from build123d import *

# Parameters (mm, degrees)
SKETCH2_W           = 50
SKETCH2_H           = 225
SKETCH2_W_2         = 30
SKETCH2_H_2         = 205
BOSS_EXTRUDE1_DEPTH = 25
SKETCH3_W           = 140
SKETCH3_H           = 305
SKETCH3_W_2         = 30
SKETCH3_H_2         = 205
BOSS_EXTRUDE2_DEPTH = 10
BOSS_EXTRUDE3_DEPTH = 150
BOSS_EXTRUDE4_START = 20
BOSS_EXTRUDE4_DEPTH = 5
LPATTERN1_COUNT     = 6
LPATTERN1_PITCH     = 22


with BuildPart() as part:
    # Sketch2 → Boss-Extrude1 (new body)
    with BuildSketch(Plane.XY):
        Rectangle(SKETCH2_W, SKETCH2_H)
        Rectangle(SKETCH2_W_2, SKETCH2_H_2, mode=Mode.SUBTRACT)
    extrude(amount=-BOSS_EXTRUDE1_DEPTH)

    # Sketch3 → Boss-Extrude2 (add)
    with BuildSketch(Plane.XY):
        with Locations((15, 0)):
            Rectangle(SKETCH3_W, SKETCH3_H)
        Rectangle(SKETCH3_W_2, SKETCH3_H_2, mode=Mode.SUBTRACT)
    extrude(amount=BOSS_EXTRUDE2_DEPTH)

    # Sketch4 → Boss-Extrude3 (add)
    with BuildSketch(Plane.XY.offset(10)):
        with BuildLine():
            Line((-30, 137.5), (65, 137.5))
            ThreePointArc((65, 137.5), (75.606601718, 133.106601718), (80, 122.5))
            Line((80, 122.5), (80, -122.5))
            ThreePointArc((80, -122.5), (75.606601718, -133.106601718), (65, -137.5))
            Line((65, -137.5), (-30, -137.5))
            ThreePointArc((-30, -137.5), (-40.606601718, -133.106601718), (-45, -122.5))
            Line((-45, -122.5), (-45, 122.5))
            ThreePointArc((-45, 122.5), (-40.606601718, 133.106601718), (-30, 137.5))
        make_face()
        with BuildLine():
            Line((-25, 122.5), (60, 122.5))
            ThreePointArc((60, 122.5), (63.535533906, 121.035533906), (65, 117.5))
            Line((65, 117.5), (65, -117.5))
            ThreePointArc((65, -117.5), (63.535533906, -121.035533906), (60, -122.5))
            Line((60, -122.5), (-25, -122.5))
            ThreePointArc((-25, -122.5), (-28.535533906, -121.035533906), (-30, -117.5))
            Line((-30, -117.5), (-30, 117.5))
            ThreePointArc((-30, 117.5), (-28.535533906, 121.035533906), (-25, 122.5))
        make_face(mode=Mode.SUBTRACT)
    extrude(amount=BOSS_EXTRUDE3_DEPTH)

    # Sketch5 → Boss-Extrude4 (add)
    with BuildSketch(Plane.XY.offset(10).offset(BOSS_EXTRUDE4_START)):
        with BuildLine():
            Line((-35, 142.5), (70, 142.5))
            ThreePointArc((70, 142.5), (80.606601718, 138.106601718), (85, 127.5))
            Line((85, 127.5), (85, -127.5))
            ThreePointArc((85, -127.5), (80.606601718, -138.106601718), (70, -142.5))
            Line((70, -142.5), (-35, -142.5))
            ThreePointArc((-35, -142.5), (-45.606601718, -138.106601718), (-50, -127.5))
            Line((-50, -127.5), (-50, 127.5))
            ThreePointArc((-50, 127.5), (-45.606601718, 138.106601718), (-35, 142.5))
        make_face()
        with BuildLine():
            Line((-30, 137.5), (65, 137.5))
            ThreePointArc((65, 137.5), (75.606601718, 133.106601718), (80, 122.5))
            Line((80, 122.5), (80, -122.5))
            ThreePointArc((80, -122.5), (75.606601718, -133.106601718), (65, -137.5))
            Line((65, -137.5), (-30, -137.5))
            ThreePointArc((-30, -137.5), (-40.606601718, -133.106601718), (-45, -122.5))
            Line((-45, -122.5), (-45, 122.5))
            ThreePointArc((-45, 122.5), (-40.606601718, 133.106601718), (-30, 137.5))
        make_face(mode=Mode.SUBTRACT)
    boss_extrude4 = extrude(amount=BOSS_EXTRUDE4_DEPTH)

    # LPattern1: Boss-Extrude4 ×6
    with Locations(*[(0, 0, i * LPATTERN1_PITCH) for i in range(1, LPATTERN1_COUNT)]):
        add(boss_extrude4)


solid = part.part
Source: CAD feature listing. Evaluate the final solid. Frame: model axes, mm. A direction names the side the tool comes from. Round coordinates to 2 decimals unless told otherwise and drop trailing zeros. Order: outer loops, then holes, each group sorted by start corner. A loop starts at its lowest first (then second) coordinate and runs counter-clockwise, first axis right, second up. Notation, with made-up numbers: (76.5, 48.25) -> (87.5, 48.25) arc R21 cw to (87.5, 66.25) -> close; hole circle Ø8 at (69.5, 71.25). An arc over 180 degrees is marked (long way). Answer as CSV lines item,"result".
Item 1: Pin query (flat end, axial travel): pin 1 Ø12 at (x, y) = (10.5, 31.5) entering from +Z; pin 2 Ø5 at (x, z) = (35.5, 62) entering from -Y; pin 3 Ø2.5 at (x, z) = (-5, 33.5) entering from +Y. Return the tip coordinate at first contact, or that it passes through.
A:
pin 1,"z = 10"
pin 2,"y = -137.5"
pin 3,"y = 142.5"
Item 2: Line query: L1, parallel to X at y = 67.5, z = -12.5; L2, parallel to Y at x = 48.5, z = 72.5; L3, parallel to Y at x = -13, z = 5. Output: solid intervals per line, ascending.
A:
L1,"-25 to -15, 15 to 25"
L2,"-137.5 to -122.5, 122.5 to 137.5"
L3,"-152.5 to -102.5, 102.5 to 152.5"
Item 3: Section A-A, the plane z = 64. Return loops of the section in (x, y).
A:
outline,"(-45, -122.5) arc R15 ccw to (-30, -137.5) -> (65, -137.5) arc R15 ccw to (80, -122.5) -> (80, 122.5) arc R15 ccw to (65, 137.5) -> (-30, 137.5) arc R15 ccw to (-45, 122.5) -> close; hole (-30, -117.5) arc R5 ccw to (-25, -122.5) -> (60, -122.5) arc R5 ccw to (65, -117.5) -> (65, 117.5) arc R5 ccw to (60, 122.5) -> (-25, 122.5) arc R5 ccw to (-30, 117.5) -> close"
Item 4: Pull-direction query (Z, two-part tool) for faces 1 (the face through (80.49, 138.22, 54.46)), 2 (the face through (83, 32, 101)); classes: pulls with the +Z half, pulls with the -Z half, needs draft (parallel to the pull), parting line crosses it, or undercut.
A:
face 1,"needs draft"
face 2,"undercut"
Item 5: Reachability of faces 3 (the face through (-40.72, 132.99, 131.38)), 4 (the face through (75.72, -132.99, 19.86)), 5 (the face through (80.49, 138.22, 32.47)), 6 (the face through (17, 137.5, 65)) from +Z, -Z, +X, -X, +Y, -Y: full face, straight path, thin tool, end or side. Return the list, or none.
A:
face 3,"-X, +Y"
face 4,"+X, -Y"
face 5,"+Z, +X, +Y"
face 6,"+X, -X, +Y"
